Check sheet for the modelled part. Datum: model origin and axes. Units: mm. Face numbers are marked on the shaded views. A direction names the side the tool comes from. Give positions to 0.01 mm unless a question says otherwise; leave off trailing zeros. Order: outer loops, then holes, each group sorted by start corner. A loop starts at its lowest first (then second) coordinate and runs counter-clockwise, first axis right, second up.
from build123d import *

# Parameters (mm, degrees)
PAD_DEPTH       = 30.5
SKETCH001_R     = 2
SKETCH001_W     = 5
SKETCH001_H     = 20
POCKET_DEPTH    = 53.001
CHAMFER_SIZE    = 2
PAD001_DEPTH    = 3
PAD002_DEPTH    = 3
SKETCH004_W     = 5
SKETCH004_H     = 20
POCKET001_DEPTH = 84.501


with BuildPart() as part:
    # Sketch → Pad (new body)
    with BuildSketch(Plane.XY):
        Polygon((0, 0), (20, 0), (20, 50), (81.5, 50), (81.5, 0), (101.5, 0), (101.5, 3), (84.5, 3), (84.5, 53), (17, 53), (17, 3), (0, 3), align=None)
    extrude(amount=PAD_DEPTH)

    # Sketch001 (on Face1 of Pad) → Pocket (cut, through all)
    with BuildSketch(Plane.XZ):
        with Locations((10, 15)):
            Circle(SKETCH001_R)
        with Locations((92.5, 15)):
            Circle(SKETCH001_R)
        with Locations((31.25, 15)):
            Rectangle(SKETCH001_W, SKETCH001_H)
        with Locations((71.25, 15)):
            Rectangle(SKETCH001_W, SKETCH001_H)
        with Locations((63.25, 15)):
            Rectangle(SKETCH001_W, SKETCH001_H)
        with Locations((39.25, 15)):
            Rectangle(SKETCH001_W, SKETCH001_H)
        with Locations((47.25, 15)):
            Rectangle(SKETCH001_W, SKETCH001_H)
        with Locations((55.25, 15)):
            Rectangle(SKETCH001_W, SKETCH001_H)
    extrude(amount=-POCKET_DEPTH, mode=Mode.SUBTRACT)

    # Chamfer
    chamfer_edges = [part.edges().sort_by_distance(p)[0] for p in [
        (90.5, 3, 15),
        (8, 3, 15),
    ]]
    chamfer(chamfer_edges, length=CHAMFER_SIZE)

    # Sketch003 (on Face6 of Chamfer) → Pad001 (join)
    with BuildSketch(Plane.XY):
        Polygon((0, 0), (20, 0), (20, 42.928932), (27.071068, 50), (74.428932, 50), (81.5, 42.928932), (81.5, 0), (101.5, 0), (101.5, 3), (91.571068, 3), (84.5, 10.071068), (84.5, 53), (17, 53), (17, 10.071068), (9.928932, 3), (0, 3), align=None)
    extrude(amount=-PAD001_DEPTH)

    # Sketch002 (on Face7 of Pad001) → Pad002 (join)
    with BuildSketch(Plane.XY.offset(30.5)):
        Polygon((0, 0), (20, 0), (20, 42.928932), (27.071068, 50), (74.428932, 50), (81.5, 42.928932), (81.5, 0), (101.5, 0), (101.5, 3), (91.571068, 3), (84.5, 10.071068), (84.5, 53), (17, 53), (17, 10.071068), (9.928932, 3), (0, 3), align=None)
    extrude(amount=PAD002_DEPTH)

    # Sketch004 (on Face75 of Pad002) → Pocket001 (cut, through all)
    with BuildSketch(Plane.YZ.offset(84.5)):
        with Locations((17.5, 15)):
            Rectangle(SKETCH004_W, SKETCH004_H)
        with Locations((25.5, 15)):
            Rectangle(SKETCH004_W, SKETCH004_H)
        with Locations((33.5, 15)):
            Rectangle(SKETCH004_W, SKETCH004_H)
        with Locations((41.5, 15)):
            Rectangle(SKETCH004_W, SKETCH004_H)
    extrude(amount=-POCKET001_DEPTH, mode=Mode.SUBTRACT)


solid = part.part
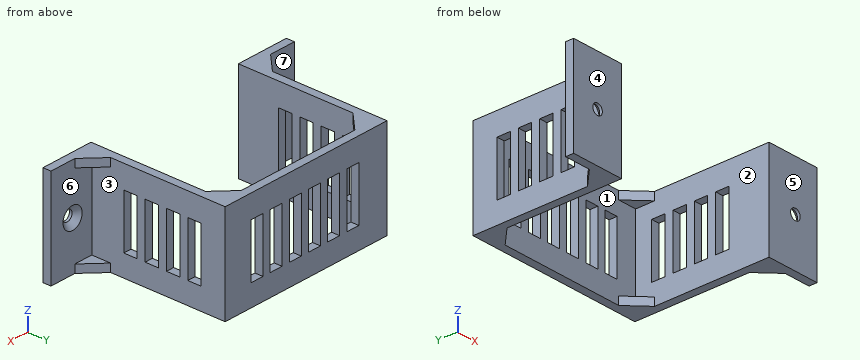
1) Depth check by flat-ended pin: pin 1 Ø6 at (x, z) = (74.5, 24.5) entering from -Y; pin 2 Ø6 at (x, y) = (76, 24) entering from -Z; pin 3 Ø13.5 at (x, z) = (95, 10) entering from +Y; pin 4 Ø2.5 at (y, z) = (51.5, 10.5) entering from +X. Enter the tip coordinate at first touch or a pass-through.
Recorded:
pin 1: stops at y = 50
pin 2: passes through
pin 3: stops at y = 3
pin 4: stops at x = 84.5
2) Section check D-D, the plane y = 34. Record the cut outline in (x, z).
Recorded:
outline: (17, -3) - (20, -3) - (20, 5) - (17, 5) - close; (17, 25) - (20, 25) - (20, 33.5) - (17, 33.5) - close; (81.5, -3) - (84.5, -3) - (84.5, 5) - (81.5, 5) - close; (81.5, 25) - (84.5, 25) - (84.5, 33.5) - (81.5, 33.5) - close
3) Draft check along X on the marked faces 1, 2, 3 and 4. Enter one of: +X half, -X half, draft (parallel to the pull), parting line (faces both ways), or undercut.
Recorded:
face 1: undercut
face 2: undercut
face 3: +X half
face 4: draft
4) Section check A-A, the plane x = 83.5. Record the cut outline in (y, z), then the cut area to 3 significant figures.
Recorded:
outline: (0, -3) - (53, -3) - (53, 33.5) - (0, 33.5) - close; hole (15, 5) - (20, 5) - (20, 25) - (15, 25) - close; hole (23, 5) - (28, 5) - (28, 25) - (23, 25) - close; hole (31, 5) - (36, 5) - (36, 25) - (31, 25) - close; hole (39, 5) - (44, 5) - (44, 25) - (39, 25) - close
area: 1,530 mm2
5) Section check C-C, the plane y = 11.5. Record the cut outline in (x, z).
Recorded:
outline: (17, -3) - (20, -3) - (20, 33.5) - (17, 33.5) - close; (81.5, -3) - (84.5, -3) - (84.5, 33.5) - (81.5, 33.5) - close
6) Material ranges on L1, parallel to Y at x = 83.5, z = 15; L2, parallel to Z at x = 92.5, y = 0.25; L3, parallel to X at y = 9.5, z = 11, recorded low to high.
Recorded:
L1: y = 0 to 15, 20 to 23, 28 to 31, 36 to 39, 44 to 53
L2: z = -3 to 13, 17 to 33.5
L3: x = 17 to 20, 81.5 to 84.5
7) Set-up check for the marked faces 5, 6 and 7: record each of +Z, -Z, +X, -X, +Y, -Y from which the full face is reachable in a straight line by a thin tool's end or side.
Recorded:
face 5: +Z, -Z, +X, -X, -Y
face 6: +X, +Y
face 7: -X, +Y
8) Section check B-B, the plane z = 27.5. Record the cut outline in (x, y).
Recorded:
outline: (0, 0) - (20, 0) - (20, 50) - (81.5, 50) - (81.5, 0) - (101.5, 0) - (101.5, 3) - (84.5, 3) - (84.5, 53) - (17, 53) - (17, 3) - (0, 3) - close
